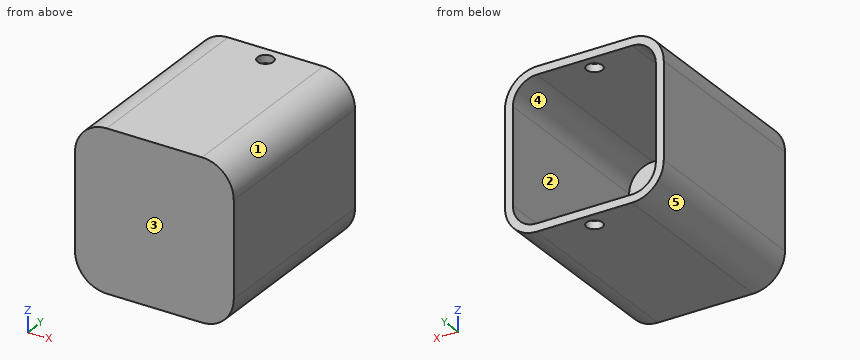
from build123d import *

# Parameters (mm, degrees)
SKETCH1_W           = 50
SKETCH1_H           = 50
BOSS_EXTRUDE1_DEPTH = 60
FILLET1_R           = 10
SHELL1_T            = -2.5
SKETCH2_R           = 2.5
CUT_EXTRUDE1_DEPTH  = 93.736184955


with BuildPart() as part:
    # Sketch1 → Boss-Extrude1 (new body)
    with BuildSketch(Plane(origin=(0, 0, 0), x_dir=(1, 0, 0), z_dir=(0, 1, 0))):
        with Locations((25, 25)):
            Rectangle(SKETCH1_W, SKETCH1_H)
    extrude(amount=BOSS_EXTRUDE1_DEPTH)

    # Fillet1
    fillet1_edges = [part.edges().sort_by_distance(p)[0] for p in [
        (0, 30, -50),
        (50, 30, -50),
        (50, 30, 0),
        (0, 30, 0),
    ]]
    fillet(fillet1_edges, radius=FILLET1_R)

    # Shell1
    shell1_openings = [part.faces().sort_by_distance(p)[0] for p in [
        (25, 60, -25),
    ]]
    offset(amount=SHELL1_T, openings=shell1_openings, kind=Kind.INTERSECTION)

    # Sketch2 → Cut-Extrude1 (cut, through all)
    with BuildSketch(Plane.XY):
        with Locations((25, 55)):
            Circle(SKETCH2_R)
    extrude(amount=-CUT_EXTRUDE1_DEPTH, mode=Mode.SUBTRACT)


solid = part.part
Could you check a few things on this model? Use its own coordinates, in mm. Face numbers are marked on the shaded views. A direction names the side the tool comes from. Coordinates: 2 decimals unless noted, no trailing zeros. Order: outer loops, then holes, each group sorted by start corner. A loop starts at its lowest first (then second) coordinate and runs counter-clockwise, first axis right, second up.
Q1. Suppose I cut it at D-D on x = 39. Please give me the cut outline in (y, z).
Q2. Suppose I cut it at B-B on x = 25. Please give me the cut outline in (y, z), and give its area (4 significant figures).
Q3. Will these pins go through, and if not, where does the flat tip stop? pin 1 (6 mm diameter, centred on x = 43, z = -13, fed in from +Y); pin 2 (4.5 mm diameter, centred on x = 25, y = 55, fed in from -Z).
Q4. Suppose I cut it at C-C on y = 23. Please give me the cut outline in (x, z), and give its area (3 significant figures).
Q5. Please list where these lines run through material, in increasing order: L1, parallel to Z at x = 9.5, y = 52.5; L2, parallel to Y at x = 25, z = -0.5; L3, parallel to X at y = 39, z = -34.
Q6. Thinking about a two-plate mould opening in Z: for the marked faces 1, 2 and 3, which applies, released by +Z, released by -Z, zero draft, split by the parting line, or undercut?
Q7. Suppose I cut it at A-A on y = 53.5. Please give me the cut outline in (x, z).
Q8. Which directions (+Z, -Z, +X, -X, +Y, -Y) give clear straight access to the entire face, cutting with the end or side of a thin tool? Please do the marked faces 4 and 5.
Answer:
1. outline: (0, -50) - (60, -50) - (60, -47.5) - (2.5, -47.5) - (2.5, -2.5) - (60, -2.5) - (60, 0) - (0, 0) - close
2. outline: (0, -50) - (52.5, -50) - (52.5, -47.5) - (2.5, -47.5) - (2.5, -2.5) - (52.5, -2.5) - (52.5, 0) - (0, 0) - close; (57.5, -50) - (60, -50) - (60, -47.5) - (57.5, -47.5) - close; (57.5, -2.5) - (60, -2.5) - (60, 0) - (57.5, 0) - close
2. area: 387.5 mm2
3. pin 1: stops at y = 2.5
3. pin 2: passes through
4. outline: (0, -40) arc R10 ccw to (10, -50) - (40, -50) arc R10 ccw to (50, -40) - (50, -10) arc R10 ccw to (40, 0) - (10, 0) arc R10 ccw to (0, -10) - close; hole (2.5, -40) arc R7.5 ccw to (10, -47.5) - (40, -47.5) arc R7.5 ccw to (47.5, -40) - (47.5, -10) arc R7.5 ccw to (40, -2.5) - (10, -2.5) arc R7.5 ccw to (2.5, -10) - close
4. area: 437 mm2
5. L1: z = -49.99 to -47.48, -2.52 to -0.01
5. L2: y = 0 to 52.5, 57.5 to 60
5. L3: x = 0 to 2.5, 47.5 to 50
6. face 1: released by +Z
6. face 2: undercut
6. face 3: zero draft
7. outline: (0, -40) arc R10 ccw to (10, -50) - (23, -50) - (23, -47.5) - (10, -47.5) arc R7.5 cw to (2.5, -40) - (2.5, -10) arc R7.5 cw to (10, -2.5) - (23, -2.5) - (23, 0) - (10, 0) arc R10 ccw to (0, -10) - close; (27, -50) - (40, -50) arc R10 ccw to (50, -40) - (50, -10) arc R10 ccw to (40, 0) - (27, 0) - (27, -2.5) - (40, -2.5) arc R7.5 cw to (47.5, -10) - (47.5, -40) arc R7.5 cw to (40, -47.5) - (27, -47.5) - close
8. face 4: +Y
8. face 5: -Z, -X, +Y, -Y
